The listing builds one solid part. Answer for the finished solid, in the listing's coordinates (mm). Face numbers are marked on the shaded views. A direction names the side the tool comes from. Give positions to 0.01 mm unless a question says otherwise; leave off trailing zeros. Loops run counter-clockwise (first coordinate to the right, second up) from the corner with the lowest first, then second, coordinate; pieces in that order, holes last. Notation, with made-up numbers: (37, 23) - (57, 23) arc R12 ccw to (57, 38) - close; hole circle Ø5 at (30.5, -8.5). An arc over 180 degrees is marked (long way). Answer as CSV lines item,"result". Start each with the question number.
1) A cutting plane is placed at A-A (x = -86). Determine the outline of the cut face in (y, z).
2) For the marked faces 1 and 2, determine the directions among +Z, -Z, +X, -X, +Y, -Y from which every point of the face is accessible in a straight line to the end or side of a thin tool.
3) A cutting plane is placed at D-D (z = 18.25). Determine the outline of the cut face in (x, y), and give its area (3 significant figures).
4) For a pull along X with two mould halves and no side action, classify the marked faces 3, 4 and 5 as pulls with the +X half, pulls with the -X half, needs draft (parallel to the pull), parting line crosses it, or undercut.
5) A cutting plane is placed at C-C (y = -4). Determine the outline of the cut face in (x, z), and give its area (3 significant figures).
6) Flat-ended cylindrical pins translate along their axes: pin 1 (4 mm diameter, centred on x = -106, y = 80, fed in from +Z); pin 2 (3.5 mm diameter, centred on x = -111.5, y = 104.25, fed in from +Z); pin 3 (5 mm diameter, centred on x = -111.5, y = 27.75, fed in from -Z); pin 4 (3 mm diameter, centred on x = -98, y = 88, fed in from +Z). Find the tip coordinate at first contact, or state that the pin passes through.
7) A cutting plane is placed at B-B (x = -75). Determine the outline of the cut face in (y, z), and give its area (3 significant figures).
8) Find the intervals of material crossed by line 1 along Y through (x, z) = (-75, 4.75); line 2 along Y through (x, z) = (-60.5, 27.2); line 3 along X through (y, z) = (42.5, 6), in increasing order.
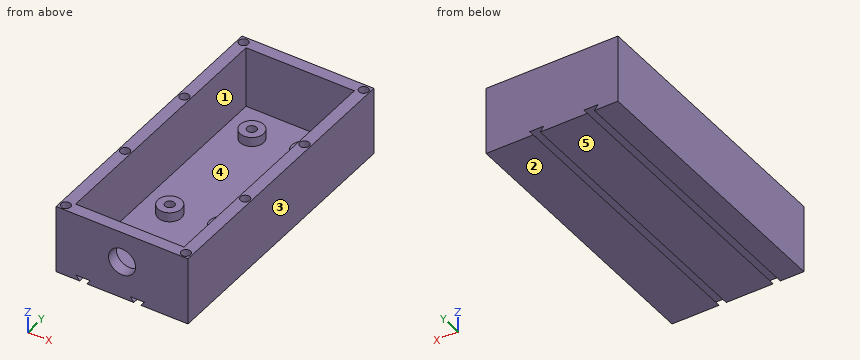
```python
from build123d import *

# Parameters (mm, degrees)
SKICA1_W                      = 56
SKICA1_H                      = 120
P_IDAT_VYSUNUT_M1_DEPTH       = 3
SKICA2_W                      = 56
SKICA2_H                      = 120
SKICA2_W_2                    = 46
SKICA2_H_2                    = 110
P_IDAT_VYSUNUT_M2_DEPTH       = 26
SKICA3_R                      = 5.75
ODEBRAT_VYSUNUT_M1_DEPTH      = 5
SKICA4_R                      = 5
SKICA4_R_2                    = 2
P_IDAT_VYSUNUT_M3_DEPTH       = 4
SKICA5_R                      = 2
ODEBRAT_VYSUNUT_M2_DEPTH      = 4
ODEBRAT_VYSUNUT_M3_DEPTH      = 169.038686022
ODEBRAT_VYSUNUT_M3_DEPTH_BACK = 169.038686022


with BuildPart() as part:
    # Skica1 → P_idat vysunut_m1 (new body)
    with BuildSketch(Plane.XY):
        with Locations((-86, 47)):
            Rectangle(SKICA1_W, SKICA1_H)
    extrude(amount=P_IDAT_VYSUNUT_M1_DEPTH)



with BuildPart() as body_2:
    # Skica2 → P_idat vysunut_m2 (new body)
    with BuildSketch(Plane.XY.offset(3)):
        with Locations((-86, 47)):
            Rectangle(SKICA2_W, SKICA2_H)
        with Locations((-86, 47)):
            Rectangle(SKICA2_W_2, SKICA2_H_2, mode=Mode.SUBTRACT)
    extrude(amount=P_IDAT_VYSUNUT_M2_DEPTH)

    # Skica3 → Odebrat vysunut_m1 (cut)
    with BuildSketch(Plane.XZ.offset(13)):
        with Locations(Location((-86, 16, 0), (0, 0, 270))):
            Circle(SKICA3_R)
    extrude(amount=-ODEBRAT_VYSUNUT_M1_DEPTH, mode=Mode.SUBTRACT)


with BuildPart() as part_1:
    add(part.part)

    add(body_2.part)  # P_idat vysunut_m3 merges body 2
    # Skica4 → P_idat vysunut_m3 (add)
    # profile 1 of 4: a face of its own
    with BuildSketch(Plane.XY.offset(3)):
        with Locations((-97, 87.5)):
            Circle(SKICA4_R)
        with Locations((-97, 87.5)):
            Circle(SKICA4_R_2, mode=Mode.SUBTRACT)
    # profile 2 of 4: a face of its own
    with BuildSketch(Plane.XY.offset(3)):
        with Locations((-97, 34.5)):
            Circle(SKICA4_R)
        with Locations((-97, 34.5)):
            Circle(SKICA4_R_2, mode=Mode.SUBTRACT)
    # profile 3 of 4: a face of its own
    with BuildSketch(Plane.XY.offset(3)):
        with Locations(Location((-75, 34.5, 0), (0, 0, 180))):
            Circle(SKICA4_R)
        with Locations(Location((-75, 34.5, 0), (0, 0, 180))):
            Circle(SKICA4_R_2, mode=Mode.SUBTRACT)
    # profile 4 of 4: a face of its own
    with BuildSketch(Plane.XY.offset(3)):
        with Locations(Location((-75, 87.5, 0), (0, 0, 180))):
            Circle(SKICA4_R)
        with Locations(Location((-75, 87.5, 0), (0, 0, 180))):
            Circle(SKICA4_R_2, mode=Mode.SUBTRACT)
    extrude(amount=P_IDAT_VYSUNUT_M3_DEPTH)

    # Skica5 → Odebrat vysunut_m2 (cut)
    with BuildSketch(Plane.XY.offset(29)):
        with Locations((-111.5, -10.5)):
            Circle(SKICA5_R)
        with Locations((-60.5, -10.5)):
            Circle(SKICA5_R)
        with Locations((-60.5, 27.75)):
            Circle(SKICA5_R)
        with Locations((-60.5, 66)):
            Circle(SKICA5_R)
        with Locations((-60.5, 104.25)):
            Circle(SKICA5_R)
        with Locations((-111.5, 27.75)):
            Circle(SKICA5_R)
        with Locations((-111.5, 66)):
            Circle(SKICA5_R)
        with Locations((-111.5, 104.25)):
            Circle(SKICA5_R)
    extrude(amount=-ODEBRAT_VYSUNUT_M2_DEPTH, mode=Mode.SUBTRACT)

    # Skica6 → Odebrat vysunut_m3 (cut, two sides: drawn at the far end of the back side and taken through both)
    with BuildSketch(Plane(origin=(0, 107, 0), x_dir=(1, 0, 0), z_dir=(0, 1, 0)).offset(-ODEBRAT_VYSUNUT_M3_DEPTH_BACK)):
        Polygon((-104, 0), (-105.5, -2), (-99.5, -2), (-101, 0), align=None)
        Polygon((-81, 0), (-82.5, -2), (-76.5, -2), (-78, 0), align=None)
    extrude(amount=ODEBRAT_VYSUNUT_M3_DEPTH + ODEBRAT_VYSUNUT_M3_DEPTH_BACK, mode=Mode.SUBTRACT)


solid = part_1.part
```
Ans:
1,outline,"(-13, 0) - (107, 0) - (107, 29) - (102, 29) - (102, 3) - (-8, 3) - (-8, 10.25) - (-13, 10.25) - close; (-13, 21.75) - (-8, 21.75) - (-8, 29) - (-13, 29) - close"
2,face 1,"+Z"
2,face 2,"-Z, +X, -X, +Y, -Y"
3,outline,"(-114, -13) - (-91.29, -13) - (-91.29, -8) - (-109, -8) - (-109, 102) - (-63, 102) - (-63, -8) - (-80.71, -8) - (-80.71, -13) - (-58, -13) - (-58, 107) - (-114, 107) - close"
3,area,"1,610 mm2"
4,face 3,"pulls with the +X half"
4,face 4,"undercut"
4,face 5,"needs draft"
5,outline,"(-114, 0) - (-104, 0) - (-105.5, 2) - (-99.5, 2) - (-101, 0) - (-81, 0) - (-82.5, 2) - (-76.5, 2) - (-78, 0) - (-58, 0) - (-58, 29) - (-63, 29) - (-63, 3) - (-109, 3) - (-109, 29) - (-114, 29) - close"
5,area,"410 mm2"
6,pin 1,"z = 3"
6,pin 2,"z = 25"
6,pin 3,"z = 0"
6,pin 4,"z = 7"
7,outline,"(-13, 0) - (107, 0) - (107, 29) - (102, 29) - (102, 3) - (92.5, 3) - (92.5, 7) - (89.5, 7) - (89.5, 3) - (85.5, 3) - (85.5, 7) - (82.5, 7) - (82.5, 3) - (39.5, 3) - (39.5, 7) - (36.5, 7) - (36.5, 3) - (32.5, 3) - (32.5, 7) - (29.5, 7) - (29.5, 3) - (-8, 3) - (-8, 29) - (-13, 29) - close"
7,area,"668 mm2"
8,line 1,"-13 to -8, 29.5 to 32.5, 36.5 to 39.5, 82.5 to 85.5, 89.5 to 92.5, 102 to 107"
8,line 2,"-13 to -12.5, -8.5 to 25.75, 29.75 to 64, 68 to 102.25, 106.25 to 107"
8,line 3,"-114 to -109, -63 to -58"
